Check sheet for the modelled part. Datum: model origin and axes. Units: mm. A direction names the side the tool comes from. Give positions to 0.01 mm unless a question says otherwise; leave off trailing zeros. Write each loop counter-clockwise with the first axis right and the second up, starting at its lowest first coordinate (ties: lowest second). Pieces come first, ordered by that corner, then holes. Notation, with made-up numbers: M -4.5,-25 L 15.5,-25 A9 cw 15.5,-12 Z; hole C 25,53 d5. An arc over 180 degrees is marked long. Write item = value, one per line. Start each with the question number.
1) Gauge pin test, flat ends, axial feed: pin 1 (23 mm diameter, centred on x = 1.5, y = 59, fed in from +Z); pin 2 (12 mm diameter, centred on y = 9, z = 37.5, fed in from -X); pin 3 (7.5 mm diameter, centred on y = 17, z = 4, fed in from -X). Record the tip position at first contact, or that the pin passes through.
2) Sectioned sample at D-D, the plane z = 8. Record the cut outline in (x, y).
3) Draft check along X on faces 1 (the face through (13, 12, 47)), 2 (the face through (-0.96, 39.5, 3.45)), 3 (the face through (16.908, 28.346, 3.451)), 4 (the face through (14.071, 79.206, 3.451)). Enter one of: pulls with the +X half, pulls with the -X half, needs draft (parallel to the pull), parting line crosses it, or undercut.
4) Sectioned sample at A-A, the plane y = 35. Record the cut outline in (x, z).
5) Set-up check for faces 5 (the face through (26.895, 20, 3)), 6 (the face through (20.376, 9.127, 26.72)), 7 (the face through (0, 21, 3)): record each of +Z, -Z, +X, -X, +Y, -Y from which the full face is reachable in a straight line by a thin tool's end or side.
6) Sectioned sample at B-B, the plane x = 8.5. Record the cut outline in (y, z).
7) Scan lines: L1, parallel to Z at x = 30.5, y = 55; L2, parallel to X at y = 69, z = 6; L3, parallel to X at y = 55, z = 6.5. Record each from-to range of solid material in increasing order.
8) Sectioned sample at C-C, the plane y = 12. Record the cut outline in (x, z).
from build123d import *

# Parameters (mm, degrees)
SKETCH2_R           = 7.5
BOSS_EXTRUDE5_DEPTH = 7
SKETCH3_R           = 7.5
BOSS_EXTRUDE6_DEPTH = 40


with BuildPart() as part:
    # Sketch2 → Boss-Extrude5 (new body)
    with BuildSketch(Plane.XY):
        with BuildLine():
            Line((5, 0), (21.89510984, 0))
            ThreePointArc((21.89510984, 0), (25.430643746, 1.464466094), (26.89510984, 5))
            Line((26.89510984, 5), (26.89510984, 35.958548116))
            ThreePointArc((26.89510984, 35.958548116), (27.832932013, 39.458548116), (30.39510984, 42.020725942))
            Line((30.39510984, 42.020725942), (49.440130583, 53.016373795))
            ThreePointArc((49.440130583, 53.016373795), (51.323745621, 55.522595335), (50.821570497, 58.61726368))
            ThreePointArc((50.821570497, 58.61726368), (13.44755492, 79.210770001), (-23.926460657, 58.61726368))
            ThreePointArc((-23.926460657, 58.61726368), (-24.428635781, 55.522595335), (-22.545020743, 53.016373795))
            Line((-22.545020743, 53.016373795), (-3.5, 42.020725942))
            ThreePointArc((-3.5, 42.020725942), (-0.937822174, 39.458548116), (0, 35.958548116))
            Line((0, 35.958548116), (0, 5))
            ThreePointArc((0, 5), (1.464466094, 1.464466094), (5, 0))
        make_face()
        with Locations((13.44755492, 35)):
            Circle(SKETCH2_R, mode=Mode.SUBTRACT)
    extrude(amount=BOSS_EXTRUDE5_DEPTH)

    # Sketch3 → Boss-Extrude6 (add)
    with BuildSketch(Plane.XY.offset(7)):
        with Locations((13.44755492, 12)):
            Circle(SKETCH3_R)
    extrude(amount=BOSS_EXTRUDE6_DEPTH)


solid = part.part
Data:
q1.pin_1 = 7
q1.pin_2 = 5.95
q1.pin_3 = 0
q2.outline = C 13.45,12 d15
q3.face_1 = needs draft
q3.face_2 = pulls with the -X half
q3.face_3 = undercut
q3.face_4 = parting line crosses it
q4.outline = M 0,0 L 5.95,0 L 5.95,7 L 0,7 Z; M 20.95,0 L 26.9,0 L 26.9,7 L 20.95,7 Z
q5.face_5 = +Z, -Z, +X, -Y
q5.face_6 = +Z
q5.face_7 = +Z, -Z, -X, -Y
q6.outline = M 0,0 L 29.36,0 L 29.36,7 L 17.64,7 L 17.64,47 L 6.36,47 L 6.36,7 L 0,7 Z; M 40.64,0 L 78.93,0 L 78.93,7 L 40.64,7 Z
q7.L1 = 0 to 7
q7.L2 = -14.81 to 41.71
q7.L3 = -24.26 to 51.16
q8.outline = M 0,0 L 26.9,0 L 26.9,7 L 20.95,7 L 20.95,47 L 5.95,47 L 5.95,7 L 0,7 Z
